```python
from build123d import *

# Parameters (mm, degrees)
SKETCH1_W                = 30
SKETCH1_H                = 15
SKETCH1_R                = 2
BOSS_EXTRUDE1_DEPTH      = 2.5
BOSS_EXTRUDE2_DEPTH      = 10
BOSS_EXTRUDE2_DEPTH_BACK = 2.5
SKETCH1_3_R              = 2
SKETCH2_R                = 1
CUT_EXTRUDE1_DEPTH       = 10


with BuildPart() as part:
    # Sketch1 → Boss-Extrude1 (new, symmetric)
    with BuildSketch(Plane(origin=(0, 0, 0), x_dir=(1, 0, 0), z_dir=(0, 1, 0))):
        Rectangle(SKETCH1_W, SKETCH1_H)
        with Locations(Location((-5, 2.5, 0), (0, 0, 270))):
            Circle(SKETCH1_R, mode=Mode.SUBTRACT)
        with Locations(Location((-11, 0, 0), (0, 0, 270))):
            Circle(SKETCH1_R, mode=Mode.SUBTRACT)
    extrude(amount=BOSS_EXTRUDE1_DEPTH, both=True)

    # Sketch1_3 → Boss-Extrude2 (add, two sides: drawn at the far end of the back side and taken through both)
    with BuildSketch(Plane(origin=(0, 0, 0), x_dir=(1, 0, 0), z_dir=(0, 1, 0)).offset(-BOSS_EXTRUDE2_DEPTH_BACK)):
        with Locations(Location((-5, 2.5, 0), (0, 0, 270))):
            Circle(SKETCH1_3_R)
    extrude(amount=BOSS_EXTRUDE2_DEPTH + BOSS_EXTRUDE2_DEPTH_BACK)

    # Sketch2 → Cut-Extrude1 (cut)
    with BuildSketch(Plane(origin=(15, 0, 0), x_dir=(0, 0, -1), z_dir=(1, 0, 0))):
        Circle(SKETCH2_R)
    extrude(amount=-CUT_EXTRUDE1_DEPTH, mode=Mode.SUBTRACT)


solid = part.part
```
Design review of the part built by this model. Coordinates are the model's own, in mm. A direction names the side the tool comes from. Coordinates: 2 decimals unless noted, no trailing zeros. Loops run counter-clockwise (first coordinate to the right, second up) from the corner with the lowest first, then second, coordinate; pieces in that order, holes last.
Q1. To check wall thickness, follow line 1 (X direction, y = 0.5, z = 0); line 2 (X direction, y = 1.15, z = 0); line 3 (Y direction, x = 12.5, z = 0). State the ranges of each line that lie inside material, in increasing order.
Reported:
line 1: x = -15 to -13, -9 to 5
line 2: x = -15 to -13, -9 to 15
line 3: y = -2.5 to -1, 1 to 2.5
Q2. We need section A-A on x = -11. State the section outline as (y, z) points, and give its area (3 significant figures).
Reported:
outline: (-2.5, -7.5) - (2.5, -7.5) - (2.5, -2) - (-2.5, -2) - close; (-2.5, 2) - (2.5, 2) - (2.5, 7.5) - (-2.5, 7.5) - close
area: 55.0 mm2
Q3. For pin 1 (6 mm diameter, centred on x = 0, z = 2.5, fed in from +Y); pin 2 (0.6 mm diameter, centred on y = 0, z = 0, fed in from +X), all flat-tipped, find the tip position at first contact; note any pin that passes through.
Reported:
pin 1: stops at y = 2.5
pin 2: stops at x = 5
Q4. We need section C-C on y = 0. State the section outline as (x, z) points, and give its area (3 significant figures).
Reported:
outline: (-15, -7.5) - (15, -7.5) - (15, -1) - (5, -1) - (5, 1) - (15, 1) - (15, 7.5) - (-15, 7.5) - close; hole circle Ø4 at (-11, 0)
area: 417 mm2
Q5. We need section B-B on z = 0. State the section outline as (x, y) points, and give its area (3 significant figures).
Reported:
outline: (-15, -2.5) - (-13, -2.5) - (-13, 2.5) - (-15, 2.5) - close; (-9, -2.5) - (15, -2.5) - (15, -1) - (5, -1) - (5, 1) - (15, 1) - (15, 2.5) - (-9, 2.5) - close
area: 110 mm2
Q6. The part is to be moulded in two halves that separate along Y. For faces 1 (the face through (0, 2.5, 0)), 2 (the face through (-6.952, 6.198, -2.934)), 3 (the face through (5, 0, 0)), say which applies: +Y half, -Y half, draft (parallel to the pull), parting line (faces both ways), or undercut.
Reported:
face 1: +Y half
face 2: draft
face 3: undercut
Q7. We need section D-D on x = -5. State the section outline as (y, z) points.
Reported:
outline: (-2.5, -7.5) - (2.5, -7.5) - (2.5, -4.5) - (10, -4.5) - (10, -0.5) - (2.5, -0.5) - (2.5, 7.5) - (-2.5, 7.5) - close
Q8. Tool access review of faces 4 (the face through (-5, 10, -3)), 5 (the face through (10, -1, 0)): name each direction out of +Z, -Z, +X, -X, +Y, -Y from which nothing blocks a thin tool from reaching the whole face with its end or side.
Reported:
face 4: +Z, -Z, +X, -X, +Y
face 5: +X
